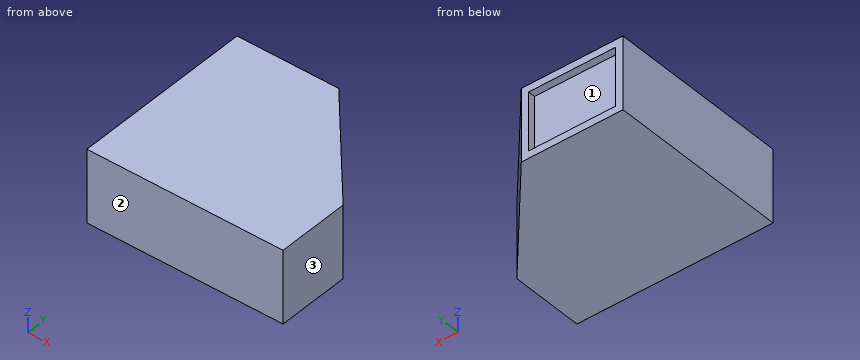
from build123d import *

# Parameters (mm, degrees)
BOSS_EXTRUDE1_DEPTH = 100
SKETCH2_W           = 120
SKETCH2_H           = 80
CUT_EXTRUDE1_DEPTH  = 10


with BuildPart() as part:
    # Sketch1 → Boss-Extrude1 (new body)
    with BuildSketch(Plane.XY):
        Polygon((135, -25), (5, 125), (-135, 125), (-135, -125), (135, -125), align=None)
    extrude(amount=BOSS_EXTRUDE1_DEPTH)

    # Sketch2 → Cut-Extrude1 (cut)
    with BuildSketch(Plane(origin=(0, 125, 0), x_dir=(1, 0, 0), z_dir=(0, 1, 0))):
        with Locations((-65, -50)):
            Rectangle(SKETCH2_W, SKETCH2_H)
    extrude(amount=-CUT_EXTRUDE1_DEPTH, mode=Mode.SUBTRACT)


solid = part.part
The listing builds one solid part. Answer for the finished solid, in the listing's coordinates (mm). Face numbers are marked on the shaded views. Coordinates: 2 decimals unless noted, no trailing zeros. Loops run counter-clockwise (first coordinate to the right, second up) from the corner with the lowest first, then second, coordinate; pieces in that order, holes last. Notation, with made-up numbers: (-13, 12) -> (27, 12) arc R10 cw to (27, 30) -> close; hole circle Ø9 at (26, 86). An arc over 180 degrees is marked (long way). Answer in a Markdown table with one row per item. Add a question column.
1. Determine the mould class of the marked faces 1, 2 and 3 for opening direction X: +X half, -X half, draft (parallel to the pull), parting line (faces both ways), or undercut.
2. Flat-ended cylindrical pins translate along their axes: P1, Ø2, axis at x = 89.5, z = 18.5, coming from the +Y side; P2, Ø3, axis at y = 119.5, z = 53, coming from the +X side; P3, Ø5, axis at x = -37.5, y = 118, coming from the -Z side; P4, Ø4, axis at x = 63, z = 83, coming from the +Y side. Find the tip coordinate at first contact, or state that the pin passes through.
3. The part is cut by section C-C, the plane y = -13. Write down the section's boundary in (x, z), then the cut area to 3 significant figures.
4. Consider line 1 (Y direction, x = -17, z = 16); line 2 (X direction, y = -2, z = 51.5); line 3 (X direction, y = 15.5, z = 30). Determine where each line is inside the solid, lowest interval first. Write a range as [from, to].
5. The part is cut by section D-D, the plane x = 116.5. Write down the section's boundary in (y, z), then the cut area to 3 significant figures.
6. The part is cut by section B-B, the plane z = 66. Write down the section's boundary in (x, y).
7. The part is cut by section A-A, the plane x = -12.5. Write down the section's boundary in (y, z), then the cut area to 3 significant figures.
Answer below:
| question | item | result |
|---|---|---|
| 1 | face 1 | undercut |
| 1 | face 2 | draft |
| 1 | face 3 | +X half |
| 2 | P1 | y = 28.65 |
| 2 | P2 | x = 11.07 |
| 2 | P3 | z = 0 |
| 2 | P4 | y = 60.38 |
| 3 | outline | (-135, 0) -> (124.6, 0) -> (124.6, 100) -> (-135, 100) -> close |
| 3 | area | 26,000 mm2 |
| 4 | line 1 | [-125, 115] |
| 4 | line 2 | [-135, 115.07] |
| 4 | line 3 | [-135, 99.9] |
| 5 | outline | (-125, 0) -> (-3.65, 0) -> (-3.65, 100) -> (-125, 100) -> close |
| 5 | area | 12,100 mm2 |
| 6 | outline | (-135, -125) -> (135, -125) -> (135, -25) -> (5, 125) -> (-5, 125) -> (-5, 115) -> (-125, 115) -> (-125, 125) -> (-135, 125) -> close |
| 7 | outline | (-125, 0) -> (125, 0) -> (125, 10) -> (115, 10) -> (115, 90) -> (125, 90) -> (125, 100) -> (-125, 100) -> close |
| 7 | area | 24,200 mm2 |
